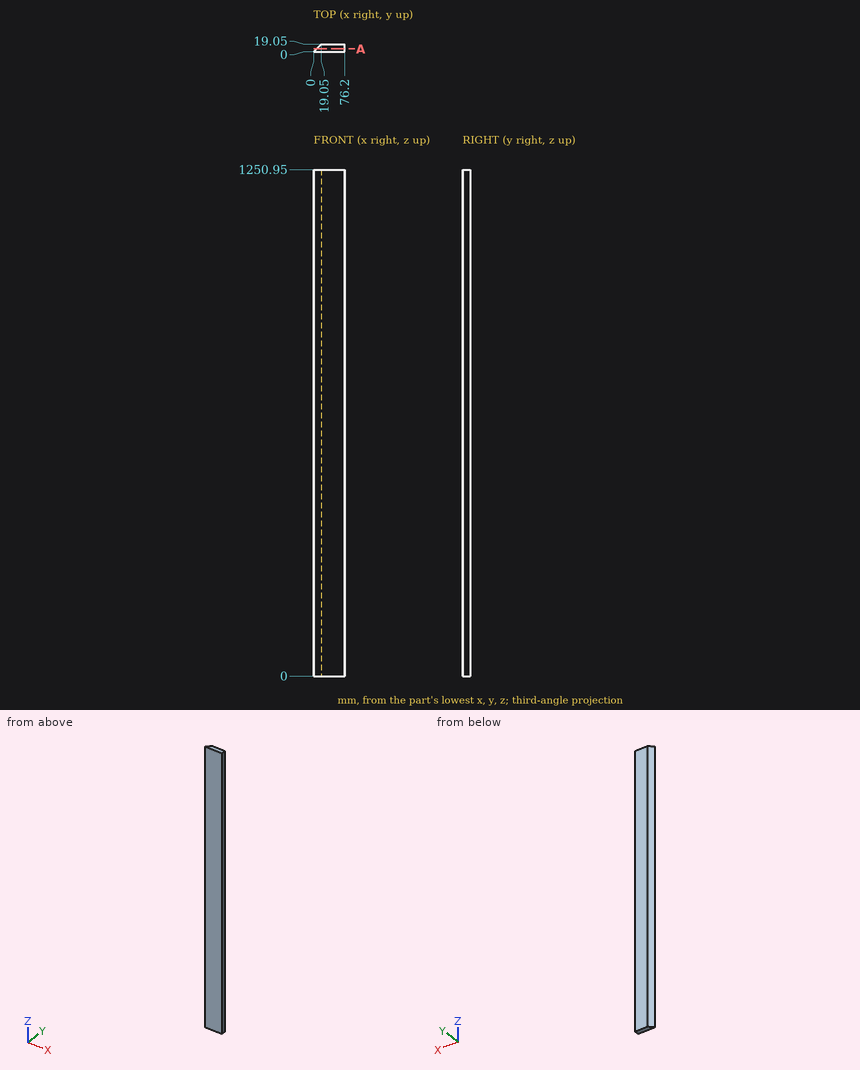
Here's the drawing with two shaded views (mm, measured from the low corner). I have some questions. Give positions to 0.01 mm unless a question says otherwise; leave off trailing zeros. Write each loop counter-clockwise with the first axis right and the second up, starting at its lowest first coordinate (ties: lowest second). Pieces come first, ordered by that corner, then holes. Notation, with made-up numbers: (-29, 26.25) -> (-12, 26.25) arc R23 cw to (-12, 55.25) -> close; hole circle Ø1 at (10, 63.25). An arc over 180 degrees is marked (long way). One line per item, written item: value.
Q1. For P1, Ø3, axis at x = 9, y = 12.5, coming from the +Z side; P2, Ø6, axis at y = 17, z = 157, coming from the -X side; P3, Ø2, axis at y = 16, z = 1022.5, coming from the -X side, each with a flat end and sliding along its axis, tell me the tip position at first contact or that it passes through.
Results found:
P1: passes through
P2: stops at x = 14
P3: stops at x = 15
Q2. Imagine slicing it at A-A on y = 7. Please give me the cut outline in (x, z).
Results found:
outline: (7, 0) -> (76.2, 0) -> (76.2, 1250.95) -> (7, 1250.95) -> close
Q3. Please list where these lines run through material, in increasing order: line 1 (X direction, y = 13.5, z = 555); line 2 (X direction, y = 6.5, z = 345.5); line 3 (Y direction, x = 13, z = 1055). Write a range as [from, to].
Results found:
line 1: x = [13.5, 76.2]
line 2: x = [6.5, 76.2]
line 3: y = [0, 13]
